from build123d import *

# Parameters (mm, degrees)
SKETCH1_R           = 2.5
BOSS_EXTRUDE2_DEPTH = 5


with BuildPart() as part:
    # Sketch1 → Boss-Extrude2 (new body)
    with BuildSketch(Plane(origin=(0, 0, 0), x_dir=(1, 0, 0), z_dir=(0, 1, 0))):
        with BuildLine():
            ThreePointArc((48.157439134, 86.819747349), (32.548521434, 75.332166703), (14.205825824, 69.075303385))
            Line((14.205825824, 69.075303385), (60.601080618, 22.857899217))
            ThreePointArc((60.601080618, 22.857899217), (66.335448138, 41.548589345), (77.473000793, 57.616563367))
            Line((77.473000793, 57.616563367), (77.416811954, 57.560374528))
            ThreePointArc((77.416811954, 57.560374528), (163.240056955, 149.970690922), (255.650373348, 235.793935922))
            ThreePointArc((255.650373348, 235.793935922), (255.754156467, 265.157091862), (226.391000527, 265.053308743))
            ThreePointArc((226.391000527, 265.053308743), (140.567755527, 172.64299235), (48.157439134, 86.819747349))
        make_face()
        with Locations(Location((53.318451782, 43.121161597, 0), (0, 0, 270))):
            Circle(SKETCH1_R, mode=Mode.SUBTRACT)
        with Locations(Location((63.9250535, 53.727763315, 0), (0, 0, 270))):
            Circle(SKETCH1_R, mode=Mode.SUBTRACT)
        with Locations(Location((33.098323122, 63.341290256, 0), (0, 0, 270))):
            Circle(SKETCH1_R, mode=Mode.SUBTRACT)
        with Locations(Location((43.70492484, 73.947891974, 0), (0, 0, 270))):
            Circle(SKETCH1_R, mode=Mode.SUBTRACT)
        with BuildLine():
            Line((55.229202732, 69.494681894), (60.091746499, 64.632138127))
            ThreePointArc((60.091746499, 64.632138127), (60.677532937, 63.217924565), (60.091746499, 61.803711002))
            Line((60.091746499, 61.803711002), (48.778038, 50.490002503))
            ThreePointArc((48.778038, 50.490002503), (47.363824438, 49.904216066), (45.949610875, 50.490002503))
            Line((45.949610875, 50.490002503), (41.087067109, 55.35254627))
            ThreePointArc((41.087067109, 55.35254627), (40.501280671, 56.766759833), (41.087067109, 58.180973395))
            Line((41.087067109, 58.180973395), (52.400775608, 69.494681894))
            ThreePointArc((52.400775608, 69.494681894), (53.81498917, 70.080468332), (55.229202732, 69.494681894))
        make_face(mode=Mode.SUBTRACT)
        Polygon((73.358826127, 72.218155358), (62.815219963, 72.218155358), (62.815219963, 82.761761522), (71.072742678, 80.475678073), align=None, mode=Mode.SUBTRACT)
        Polygon((115.901419717, 113.431281172), (104.028345777, 113.431281172), (104.028345777, 125.304355111), (121.370050098, 130.772985493), align=None, mode=Mode.SUBTRACT)
        Polygon((127.774493656, 152.369634944), (145.10497222, 154.507907615), (142.966699549, 137.177429051), (134.556556076, 134.683417686), (129.44306902, 138.846004415), (125.280482291, 143.959491471), align=None, mode=Mode.SUBTRACT)
        Polygon((161.578803014, 170.981738409), (150.580944654, 170.981738409), (150.580944654, 176.860832319), (167.661082015, 177.06401741), (167.457896924, 159.983880049), (161.578803014, 159.983880049), align=None, mode=Mode.SUBTRACT)
        Polygon((192.31024704, 206.32683153), (196.923896135, 206.32683153), (196.923896135, 201.713182434), (190.803246876, 200.206182271), align=None, mode=Mode.SUBTRACT)
        Polygon((215.737142693, 218.36823138), (208.965295985, 218.36823138), (208.965295985, 225.140078087), (215.779590379, 225.182525773), align=None, mode=Mode.SUBTRACT)
        with BuildLine():
            ThreePointArc((239.098412236, 255.098316632), (241.12410453, 255.527039925), (243.149796825, 255.098316632))
            Line((243.149796825, 255.098316632), (246.685330731, 258.633850538))
            Line((246.685330731, 258.633850538), (249.230915143, 256.088266125))
            Line((249.230915143, 256.088266125), (245.695381237, 252.552732219))
            ThreePointArc((245.695381237, 252.552732219), (246.12410453, 250.527039925), (245.695381237, 248.501347631))
            Line((245.695381237, 248.501347631), (249.230915143, 244.965813725))
            Line((249.230915143, 244.965813725), (246.685330731, 242.420229312))
            Line((246.685330731, 242.420229312), (243.149796825, 245.955763218))
            ThreePointArc((243.149796825, 245.955763218), (241.12410453, 245.527039925), (239.098412236, 245.955763218))
            Line((239.098412236, 245.955763218), (235.56287833, 242.420229312))
            Line((235.56287833, 242.420229312), (233.017293918, 244.965813725))
            Line((233.017293918, 244.965813725), (236.552827824, 248.501347631))
            ThreePointArc((236.552827824, 248.501347631), (236.12410453, 250.527039925), (236.552827824, 252.552732219))
            Line((236.552827824, 252.552732219), (233.017293918, 256.088266125))
            Line((233.017293918, 256.088266125), (235.56287833, 258.633850538))
            Line((235.56287833, 258.633850538), (239.098412236, 255.098316632))
        make_face(mode=Mode.SUBTRACT)
    extrude(amount=-BOSS_EXTRUDE2_DEPTH)


solid = part.part
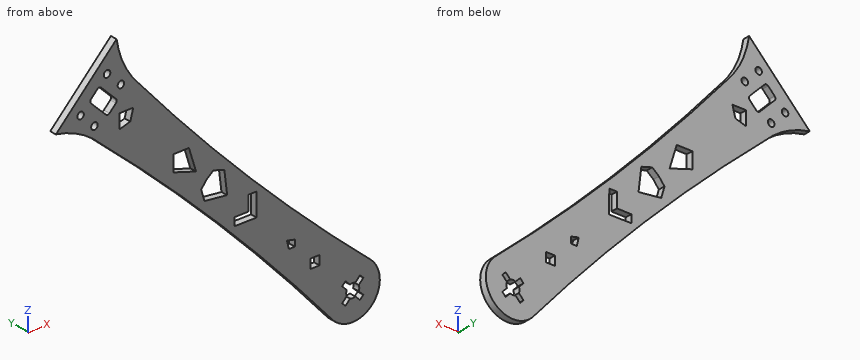
Geometry: final body of the model. Coordinates: model frame, mm. Give positions to 0.01 mm unless a question says otherwise; leave off trailing zeros. Write each loop counter-clockwise with the first axis right and the second up, starting at its lowest first coordinate (ties: lowest second). Pieces come first, ordered by that corner, then holes. Notation, with made-up numbers: M 64.25,33 L 113.25,33 A18 cw 113.25,56 Z; hole C 34,60 d4. An arc over 180 degrees is marked long. Answer in a Markdown table with one row per item. Add a question column.
(1) First-contact query: pin 1 (1.4 mm diameter, centred on y = -1.5, z = -204.5, fed in from -X); pin 2 (6.5 mm diameter, centred on x = 43.7, z = -73.95, fed in from -Y); pin 3 (1.5 mm diameter, centred on x = 110, y = -2.5, fed in from -Z); pin 4 (2.5 mm diameter, centred on x = 158.5, y = -2, fed in from -Z) (3 decimals). Flat tips, straight axial feed; report the tip coordinate or a pass-through.
(2) Section A-A on y = -1. State how many separate pieces and enclosed holes the cut face has, and give its area (3 significant figures).
(3) Section B-B on z = -91.5. Return loops of the section in (x, y), and give its area (3 significant figures).
(4) Section C-C on x = 86. Return loops of the section in (y, z).
(5) Ray query, line 1 (Z direction, x = 51.5, y = -1); line 2 (Z direction, x = 41, y = -1.5); line 3 (Z direction, x = 111, y = -0.55). Return the intervals inside material, ascending.
Result set:
| question | item | result |
|---|---|---|
| 1 | pin 1 | stops at x = 170.94 |
| 1 | pin 2 | stops at y = -5 |
| 1 | pin 3 | stops at z = -143.54 |
| 1 | pin 4 | stops at z = -192.135 |
| 2 | separate pieces | 1 |
| 2 | enclosed holes | 12 |
| 2 | area | 10,100 mm^2 |
| 3 | outline | M 53.56,-5 L 107.47,-5 L 107.47,0 L 53.56,0 Z |
| 3 | area | 270 mm^2 |
| 4 | outline | M -5,-120.44 L 0,-120.44 L 0,-67.44 L -5,-67.44 Z |
| 5 | line 1 | z = -89.71 to -68.59, -53.21 to -44.84, -41.41 to -31.92 |
| 5 | line 2 | z = -80.63 to -58.09, -55.45 to -42.38 |
| 5 | line 3 | z = -143.78 to -127.5, -113.43 to -95.37 |
